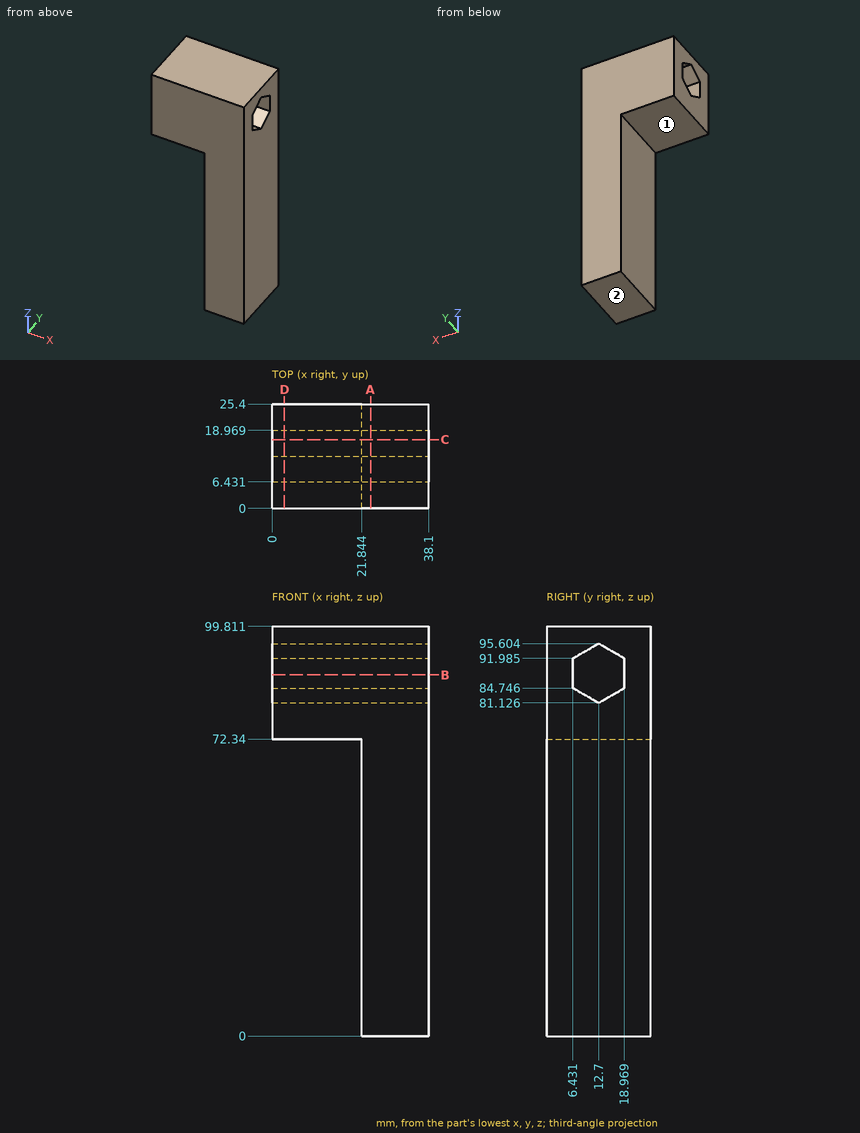
The figure shows three views and two pictorial views of one solid part (mm, origin at its lowest corner). Answer the questions. A direction names the side the tool comes from. Coordinates: 2 decimals unless noted, no trailing zeros. Loops run counter-clockwise (first coordinate to the right, second up) from the corner with the lowest first, then second, coordinate; pieces in that order, holes last.
1) Find section A-A on x = 24. Write down the section's boundary in (y, z) (1 decimal), then the cut area to 3 significant figures.
2) Flat-ended cylindrical pins translate along their axes: pin 1 Ø2 at (y, z) = (17, 57.5) entering from -X; pin 2 Ø11 at (x, y) = (6, 15.5) entering from -Z. Find the tip coordinate at first contact, or state that the pin passes through.
3) Find section B-B on z = 88. Write down the section's boundary in (x, y), then the cut area to 3 significant figures.
4) A tool of negligible diameter and unlimited length cuts with its end or side. For the marked faces 1 and 2, from which of +Z, -Z, +X, -X, +Y, -Y can it reach the whole face along a straight path? Write none if from no direction.
5) Find section C-C on y = 16.75. Write down the section's boundary in (x, z) (1 decimal).
6) Find the intervals of material crossed by L1, parallel to Z at x = 8, y = 1; L2, parallel to X at y = 16, z = 26; L3, parallel to Z at x = 8.5, y = 11 (1 decimal), in increasing order.
7) Find section D-D on x = 3. Write down the section's boundary in (y, z) (1 decimal).
Values:
1. outline: (0, 0) - (25.4, 0) - (25.4, 99.8) - (0, 99.8) - close; hole (6.4, 84.7) - (12.7, 81.1) - (19, 84.7) - (19, 92) - (12.7, 95.6) - (6.4, 92) - close
1. area: 2,400 mm2
2. pin 1: stops at x = 21.84
2. pin 2: stops at z = 72.34
3. outline: (0, 0) - (38.1, 0) - (38.1, 6.43) - (0, 6.43) - close; (0, 18.97) - (38.1, 18.97) - (38.1, 25.4) - (0, 25.4) - close
3. area: 490 mm2
4. face 1: -Z, -X, +Y, -Y
4. face 2: -Z, +X, -X, +Y, -Y
5. outline: (0, 72.3) - (21.8, 72.3) - (21.8, 0) - (38.1, 0) - (38.1, 83.5) - (0, 83.5) - close; (0, 93.3) - (38.1, 93.3) - (38.1, 99.8) - (0, 99.8) - close
6. L1: z = 72.34 to 99.81
6. L2: x = 21.84 to 38.1
6. L3: z = 72.3 to 82.1, 94.6 to 99.8
7. outline: (0, 72.3) - (25.4, 72.3) - (25.4, 99.8) - (0, 99.8) - close; hole (6.4, 84.7) - (12.7, 81.1) - (19, 84.7) - (19, 92) - (12.7, 95.6) - (6.4, 92) - close
